```python
from build123d import *

# Parameters (mm, degrees)
EXTRUDE_1_DEPTH     = 1.5
CHAMFER_1_SIZE      = 1
EXTRUDE_3_DEPTH     = 1.5
EXTRUDE_4_DEPTH     = 1.5
EXTRUDE_5_DEPTH     = 1.5
FILLET_START        = -32
FILLET_2_DEPTH      = 3
FILLET_3_R          = 0.5
SKETCH_8_W          = 30
SKETCH_8_H          = 20.8
CUT_EXTRUDE_1_DEPTH = 0.7
FILLET_4_R          = 0.5
CUT_EXTRUDE_8_DEPTH = 39.881422299


with BuildPart() as part:
    # 草图1 → 凸台-拉伸1 (new body)
    with BuildSketch(Plane.XY):
        with BuildLine():
            Line((-29.75, -1.75), (-19.75, -1.75))
            Line((-19.75, -1.75), (-9.75, -1.75))
            Line((-9.75, -1.75), (0.25, -1.75))
            ThreePointArc((0.25, -1.75), (1.310660172, -1.310660172), (1.75, -0.25))
            Line((1.75, -0.25), (1.75, 5.475))
            Line((1.75, 5.475), (1.75, 14.835))
            Line((1.75, 14.835), (1.75, 20.55))
            ThreePointArc((1.75, 20.55), (1.310660172, 21.610660172), (0.25, 22.05))
            Line((0.25, 22.05), (-9.75, 22.05))
            Line((-9.75, 22.05), (-19.75, 22.05))
            Line((-19.75, 22.05), (-29.75, 22.05))
            ThreePointArc((-29.75, 22.05), (-30.810660172, 21.610660172), (-31.25, 20.55))
            Line((-31.25, 20.55), (-31.25, 14.835))
            Line((-31.25, 14.835), (-31.25, 5.475))
            Line((-31.25, 5.475), (-31.25, -0.25))
            ThreePointArc((-31.25, -0.25), (-30.810660172, -1.310660172), (-29.75, -1.75))
        make_face()
    extrude(amount=EXTRUDE_1_DEPTH)

    # 倒角1
    chamfer_1_edges = [part.edges().sort_by_distance(p)[0] for p in [
        (-14.75, -1.75, 1.5),
        (1.310660172, -1.310660172, 1.5),
        (1.75, 10.15, 1.5),
        (1.310660172, 21.610660172, 1.5),
        (-14.75, 22.05, 1.5),
        (-31.25, 10.15, 1.5),
        (-30.810660172, 21.610660172, 1.5),
        (-30.810660172, -1.310660172, 1.5),
    ]]
    chamfer(chamfer_1_edges, length=CHAMFER_1_SIZE)

    # 草图3 → 凸台-拉伸3 (add)
    with BuildSketch(Plane(origin=(0, 22.05, 0), x_dir=(1, 0, 0), z_dir=(0, 1, 0))):
        Polygon((-19.75, -0.450892119), (-9.75, -0.450892119), (-9.75, 5), (-11.75, 7), (-17.75, 7), (-19.75, 5), align=None)
    extrude_3 = extrude(amount=-EXTRUDE_3_DEPTH)

    # 镜向1: 凸台-拉伸3 across plane
    add(extrude_3.mirror(Plane.ZX.offset(10.15)))

    # 草图4 → 凸台-拉伸4 (add)
    with BuildSketch(Plane(origin=(1.75, 0, 0), x_dir=(0, 0, -1), z_dir=(1, 0, 0))):
        Polygon((-0.4, 14.835), (5, 14.835), (7, 12.835), (7, 7.475), (5, 5.475), (-0.4, 5.475), align=None)
    extrude(amount=-EXTRUDE_4_DEPTH)

    # 草图6 → 凸台-拉伸5 (add)
    with BuildSketch(Plane.ZY.offset(31.25)):
        with BuildLine():
            Line((0.32, 14.835), (0.32, 5.475))
            Line((0.32, 5.475), (-6.88, 5.475))
            ThreePointArc((-6.88, 5.475), (-6.031471863, 5.826471863), (-5.68, 6.675))
            Line((-5.68, 6.675), (-5.68, 13.635))
            ThreePointArc((-5.68, 13.635), (-6.031471863, 14.483528137), (-6.88, 14.835))
            Line((-6.88, 14.835), (0.32, 14.835))
        make_face()
    extrude(amount=-EXTRUDE_5_DEPTH)

    # 圆角2: read off the stored shape, not the designer's step
    # 圆角2 outline → 圆角2 (cut)
    with BuildSketch(Plane.YZ.offset(FILLET_START)):
        with BuildLine():
            Line((14.835, -6.88), (14.835, -5.68))
            ThreePointArc((14.835, -5.68), (14.669164079, -5.948328157), (14.355, -5.92))
            ThreePointArc((14.355, -5.92), (14.708312629, -6.343343686), (14.835, -6.88))
        make_face()
        with BuildLine():
            ThreePointArc((5.475, -6.88), (5.601687371, -6.343343686), (5.955, -5.92))
            ThreePointArc((5.955, -5.92), (5.640835921, -5.948328157), (5.475, -5.68))
            Line((5.475, -5.68), (5.475, -6.88))
        make_face()
    extrude(amount=FILLET_2_DEPTH, mode=Mode.SUBTRACT)

    # 圆角3
    fillet_3_edges = [part.edges().sort_by_distance(p)[0] for p in [
        (-9.75, -1, 0),
        (-19.75, -1, 0),
        (-19.75, -1, -5),
        (-9.75, -1, -5),
        (-11.75, -1, -7),
        (-17.75, -1, -7),
        (1, 5.475, -5),
        (1, 14.835, 0),
        (1, 14.835, -5),
        (1, 12.835, -7),
        (1, 7.475, -7),
        (1, 5.475, 0),
        (-30.5, 14.835, 0),
        (-30.5, 5.475, 0),
        (-9.75, 21.3, 0),
        (-19.75, 21.3, 0),
        (-9.75, 21.3, -5),
        (-19.75, 21.3, -5),
        (-17.75, 21.3, -7),
        (-11.75, 21.3, -7),
    ]]
    fillet(fillet_3_edges, radius=FILLET_3_R)

    # 草图8 → 切除-拉伸1 (cut)
    with BuildSketch(Plane(origin=(0, 0, 0), x_dir=(-1, 0, 0), z_dir=(0, 0, -1))):
        with Locations((14.75, 10.15)):
            Rectangle(SKETCH_8_W, SKETCH_8_H)
    extrude(amount=-CUT_EXTRUDE_1_DEPTH, mode=Mode.SUBTRACT)

    # 圆角4
    fillet_4_edges = [part.edges().sort_by_distance(p)[0] for p in [
        (-29.75, 20.55, 0.35),
        (-29.75, -0.25, 0.35),
        (0.25, -0.25, 0.35),
        (0.25, 20.55, 0.35),
    ]]
    fillet(fillet_4_edges, radius=FILLET_4_R)

    # 草图12 → 切除-拉伸8 (cut, through all)
    with BuildSketch(Plane(origin=(0, 0, 0), x_dir=(-1, 0, 0), z_dir=(0, 0, -1))):
        with BuildLine():
            Line((1.25, 22.05), (-0.25, 22.05))
            ThreePointArc((-0.25, 22.05), (-1.310660172, 21.610660172), (-1.75, 20.55))
            Line((-1.75, 20.55), (-1.75, 19.05))
            ThreePointArc((-1.75, 19.05), (-0.871320344, 21.171320344), (1.25, 22.05))
        make_face()
        with BuildLine():
            Line((31.25, 19.05), (31.25, 20.55))
            ThreePointArc((31.25, 20.55), (30.810660172, 21.610660172), (29.75, 22.05))
            Line((29.75, 22.05), (28.25, 22.05))
            ThreePointArc((28.25, 22.05), (30.371320344, 21.171320344), (31.25, 19.05))
        make_face()
        with BuildLine():
            Line((28.25, -1.75), (29.75, -1.75))
            ThreePointArc((29.75, -1.75), (30.810660172, -1.310660172), (31.25, -0.25))
            Line((31.25, -0.25), (31.25, 1.25))
            ThreePointArc((31.25, 1.25), (30.371320344, -0.871320344), (28.25, -1.75))
        make_face()
        with BuildLine():
            Line((-1.75, 1.25), (-1.75, -0.25))
            ThreePointArc((-1.75, -0.25), (-1.310660172, -1.310660172), (-0.25, -1.75))
            Line((-0.25, -1.75), (1.25, -1.75))
            ThreePointArc((1.25, -1.75), (-0.871320344, -0.871320344), (-1.75, 1.25))
        make_face()
    extrude(amount=-CUT_EXTRUDE_8_DEPTH, mode=Mode.SUBTRACT)


solid = part.part
```
Geometry check sheet. Reference: the model listing, model coordinates, mm. A direction names the side the tool comes from. Coordinates: 2 decimals unless noted, no trailing zeros. Loops run counter-clockwise (first coordinate to the right, second up) from the corner with the lowest first, then second, coordinate; pieces in that order, holes last.
Item 1: Thickness scan on line 1 (Y direction, x = -15, z = -3.5); line 2 (X direction, y = 7.75, z = -5.5); line 3 (Z direction, x = -0.5, y = 19.5). Record the ranges inside material, lowest first.
Item 2: Sectioned sample at B-B, the plane x = -7. Record the boundary of the cut face in (y, z), then the cut area to 3 significant figures.
Item 3: Release check for a two-part mould opening along Y. For faces 1 (the face through (0.89, 21.15, 0.43)), 2 (the face through (-15, 10, 0.7)), 3 (the face through (-30.22, -0.71, 1.34)) record: released by +Y, released by -Y, zero draft, split by the parting line, or undercut.
Item 4: Sectioned sample at C-C, the plane y = 2.25. Record the boundary of the cut face in (x, z), then the cut area to 3 significant figures.
Item 5: Sectioned sample at A-A, the plane z = -2.75. Record the boundary of the cut face in (x, y) (3 decimals).
Item 6: Go/stop test with flat-tipped pins: pin 1 Ø1.6 at (x, z) = (-30.5, -2) entering from -Y (3 decimals); pin 2 Ø1.2 at (y, z) = (21.5, -2.5) entering from +X; pin 3 Ø3 at (x, y) = (-25, 3) entering from -Z. Record where each tip stops, or that it passes through.
Item 7: Access from +Z, -Z, +X, -X, +Y, -Y to the whole of each face (thin tool, end or side, straight path). Record for faces 4 (the face through (-9.75, 21, -3)), 5 (the face through (-31, 5.475, -3)), 6 (the face through (-31, 10, -5.68)), 7 (the face through (1, 14.835, -3)).
Check result:
1. line 1: y = -1.75 to -0.25, 20.55 to 22.05
1. line 2: x = -31.25 to -29.75, 0.25 to 1.75
1. line 3: z = 0.7 to 1.5
2. outline: (-1.75, 0) - (-0.25, 0) - (-0.25, 0.7) - (20.55, 0.7) - (20.55, 0) - (22.05, 0) - (22.05, 0.5) - (21.05, 1.5) - (-0.75, 1.5) - (-1.75, 0.5) - close
2. area: 20.1 mm2
3. face 1: released by +Y
3. face 2: undercut
3. face 3: released by -Y
4. outline: (-31.25, 0) - (-29.75, 0) - (-29.75, 0.7) - (0.25, 0.7) - (0.25, 0) - (1.75, 0) - (1.75, 0.5) - (0.75, 1.5) - (-30.25, 1.5) - (-31.25, 0.5) - close
4. area: 27.5 mm2
5. outline: (-31.25, 5.475) - (-29.75, 5.475) - (-29.75, 14.835) - (-31.25, 14.835) - close; (-19.75, -1.75) - (-9.75, -1.75) - (-9.75, -0.25) - (-19.75, -0.25) - close; (-19.75, 20.55) - (-9.75, 20.55) - (-9.75, 22.05) - (-19.75, 22.05) - close; (0.25, 5.475) - (1.75, 5.475) - (1.75, 14.835) - (0.25, 14.835) - close
6. pin 1: stops at y = 5.475
6. pin 2: stops at x = -9.75
6. pin 3: stops at z = 0.7
7. face 4: -Z, +X, +Y, -Y
7. face 5: -Z, +X, -X, -Y
7. face 6: -Z, -X
7. face 7: -Z, +X, -X, +Y
